CAD build for the part. Positions are in the model's coordinates, mm. A direction names the side the tool comes from. Coordinates: 2 decimals unless noted, no trailing zeros. Loops run counter-clockwise (first coordinate to the right, second up) from the corner with the lowest first, then second, coordinate; pieces in that order, holes last. Notation, with made-up numbers: (80.25, 28.5) -> (101.25, 28.5) arc R28 ccw to (101.25, 55.5) -> close; hole circle Ø11 at (9.5, 43.25). An arc over 180 degrees is marked (long way). Write item = value, one per line. Start each with the question number.
(1) Drill centre lines: line 1 (X direction, y = 49, z = 20.5); line 2 (Y direction, x = 15.24, z = 1.4); line 3 (Z direction, x = 70, y = 14.5). Where is each one in solid material? Low to high. Write a range as from..to.
(2) Pull direction X, two halves, no side cores. Call faces 1 (the face through (51.2, 50.4, 3.8)), 2 (the face through (56.89, 17.223, 6.332)), 3 (the face through (-1.252, 15.328, 59.148)): +X half, -X half, draft (parallel to the pull), parting line (faces both ways), or undercut.
(3) Band-saw the part on C-C (z = 57.15). Write the cut outline in (x, y), and give its area (3 significant figures).
(4) Band-saw the part on D-D (x = 65). Write the cut outline in (y, z) (3 decimals), and give its area (3 significant figures).
(5) Tool access for faces 4 (the face through (1.2, 51.2, 50.4)), 5 (the face through (38, 39, 2.54)), 6 (the face through (4, 10, 76.2)), 7 (the face through (30.28, 1.252, 65.576)), 8 (the face through (5.08, 33, 35)): list every direction of +Z, -Z, +X, -X, +Y, -Y with a clear straight run to the whole face (end or side of a thin tool).
(6) Band-saw the part on A-A (x = 15.24). Count the separate pieces of the cut face and the enclosed holes in it, and give its area (3 significant figures).
(7) Flat gauge pins, fed straight in: P1, Ø6.5, axis at x = 15.24, y = 57.15, coming from the +Z side; P2, Ø3, axis at x = 47.5, z = 25, coming from the +Y side; P3, Ø10, axis at y = 27.5, z = 39.5, coming from the +X side. Where does each tip first touch, or does it go through?
```python
from build123d import *

# Parameters (mm, degrees)
BOSS_EXTRUDE1_DEPTH  = 2.54
BOSS_EXTRUDE2_DEPTH  = 2.54
BOSS_EXTRUDE3_DEPTH  = 2.54
SKETCH6_W            = 2.54
SKETCH6_H            = 76.2
BOSS_EXTRUDE4_DEPTH  = 76.2
CUT_EXTRUDE1_REACH   = 133.982
SKETCH8_W            = 2.54
SKETCH8_H            = 78.74
BOSS_EXTRUDE5_DEPTH  = 76.2
CUT_EXTRUDE2_REACH   = 133.982
SKETCH10_W           = 78.74
SKETCH10_H           = 2.54
BOSS_EXTRUDE6_DEPTH  = 76.2
CUT_EXTRUDE3_REACH   = 133.982
CUT_EXTRUDE5_DEPTH   = 132.982271537
CUT_EXTRUDE6_DEPTH   = 132.982271537
CUT_EXTRUDE9_DEPTH   = 76.2
BOSS_EXTRUDE7_DEPTH  = 7.62
BOSS_EXTRUDE8_DEPTH  = 5.08
BOSS_EXTRUDE9_DEPTH  = 5.08
SKETCH34_R           = 2
CUT_EXTRUDE11_DEPTH  = 12.7
SKETCH35_R           = 2
CUT_EXTRUDE13_DEPTH  = 12.7
SKETCH36_R           = 2
CUT_EXTRUDE14_DEPTH  = 12.7
BOSS_EXTRUDE10_REACH = 133.982
SKETCH37_W           = 25.4
SKETCH37_H           = 25.4
BOSS_EXTRUDE11_REACH = 133.982
SKETCH38_W           = 25.4
SKETCH38_H           = 25.4
SKETCH39_W           = 25.4
SKETCH39_H           = 25.4
BOSS_EXTRUDE12_DEPTH = 5.08


with BuildPart() as part:
    # Sketch1 → Boss-Extrude1 (new body)
    with BuildSketch(Plane.XY):
        Polygon((0, 76.2), (0, 0), (76.2, 0), (76.2, 25.4), (25.4, 76.2), align=None)
    extrude(amount=BOSS_EXTRUDE1_DEPTH)

    # Sketch3 → Boss-Extrude2 (add)
    with BuildSketch(Plane.ZY):
        Polygon((0, 76.2), (25.4, 76.2), (76.2, 25.4), (76.2, 0), (0, 0), align=None)
    extrude(amount=BOSS_EXTRUDE2_DEPTH)

    # Sketch5 → Boss-Extrude3 (add)
    with BuildSketch(Plane.XZ):
        Polygon((-2.54, 76.2), (-2.54, 0), (76.2, 0), (76.2, 25.4), (22.86, 76.2), align=None)
    extrude(amount=BOSS_EXTRUDE3_DEPTH)

    # Sketch6 → Boss-Extrude4 (add)
    with BuildSketch(Plane.XY):
        with Locations((3.81, 38.1)):
            Rectangle(SKETCH6_W, SKETCH6_H)
    extrude(amount=BOSS_EXTRUDE4_DEPTH)

    # Sketch7 → Cut-Extrude1 (cut, up to next)
    with BuildSketch(Plane(origin=(0, 0, 0), x_dir=(0, 0, -1), z_dir=(1, 0, 0)), mode=Mode.PRIVATE) as cut_extrude1_sk1:
        Polygon((-25.4, 76.2), (-76.2, 25.4), (-76.2, 76.2), align=None)
    cut_extrude1_tool1 = extrude(cut_extrude1_sk1.sketch, amount=CUT_EXTRUDE1_REACH, mode=Mode.PRIVATE) & part.part
    add(cut_extrude1_tool1.solids().sort_by_distance((0, 59.266667, 59.266667))[0], mode=Mode.SUBTRACT)

    # Sketch8 → Boss-Extrude5 (add)
    with BuildSketch(Plane(origin=(0, 0, 0), x_dir=(0, 0, -1), z_dir=(1, 0, 0))):
        with Locations((-6.35, 36.83)):
            Rectangle(SKETCH8_W, SKETCH8_H)
    extrude(amount=BOSS_EXTRUDE5_DEPTH)

    # Sketch9 → Cut-Extrude2 (cut, up to next)
    with BuildSketch(Plane.XY, mode=Mode.PRIVATE) as cut_extrude2_sk1:
        Polygon((76.2, 25.4), (25.4, 76.2), (76.2, 76.2), align=None)
    cut_extrude2_tool1 = extrude(cut_extrude2_sk1.sketch, amount=CUT_EXTRUDE2_REACH, mode=Mode.PRIVATE) & part.part
    add(cut_extrude2_tool1.solids().sort_by_distance((59.266667, 59.266667, 0))[0], mode=Mode.SUBTRACT)

    # Sketch10 → Boss-Extrude6 (add)
    with BuildSketch(Plane.XY):
        with Locations((36.83, 3.81)):
            Rectangle(SKETCH10_W, SKETCH10_H)
    extrude(amount=BOSS_EXTRUDE6_DEPTH)

    # Sketch11 → Cut-Extrude3 (cut, up to next)
    with BuildSketch(Plane(origin=(0, 0, 0), x_dir=(1, 0, 0), z_dir=(0, 1, 0)), mode=Mode.PRIVATE) as cut_extrude3_sk1:
        Polygon((22.86, -76.2), (76.2, -25.4), (76.2, -76.2), align=None)
    cut_extrude3_tool1 = extrude(cut_extrude3_sk1.sketch, amount=CUT_EXTRUDE3_REACH, mode=Mode.PRIVATE) & part.part
    add(cut_extrude3_tool1.solids().sort_by_distance((58.42, 0, 59.266667))[0], mode=Mode.SUBTRACT)

    # Sketch12 → Cut-Extrude5 (cut, through all)
    with BuildSketch(Plane(origin=(0, 0, 0), x_dir=(0, 0, -1), z_dir=(1, 0, 0))):
        Polygon((-5.08, 5.08), (-5.08, 2.54), (-7.62, 2.54), (-7.62, 0), (-2.54, 0), (-2.54, 5.08), align=None)
    extrude(amount=CUT_EXTRUDE5_DEPTH, mode=Mode.SUBTRACT)

    # Sketch13 → Cut-Extrude6 (cut, through all)
    with BuildSketch(Plane(origin=(0, 0, 0), x_dir=(1, 0, 0), z_dir=(0, 1, 0))):
        Polygon((0, -2.54), (0, -7.62), (2.54, -7.62), (2.54, -5.08), (5.08, -5.08), (5.08, -2.54), align=None)
    extrude(amount=CUT_EXTRUDE6_DEPTH, mode=Mode.SUBTRACT)

    # Sketch15 → Cut-Extrude9 (cut)
    with BuildSketch(Plane.XY.offset(2.54)):
        Polygon((2.54, 5.08), (0, 5.08), (0, 0), (5.08, 0), (5.08, 2.54), (2.54, 2.54), align=None)
    extrude(amount=CUT_EXTRUDE9_DEPTH, mode=Mode.SUBTRACT)


with BuildPart() as cut_extrude9_piece_1:
    # of the separate pieces the step leaves, piece 1, a body of its own (cut_extrude9_pieces)
    add(part.part.solids().sort_by_distance((0, 0, 2.54))[0])



with BuildPart() as cut_extrude9_piece_2:
    # of the separate pieces the step leaves, piece 2, a body of its own (cut_extrude9_pieces)
    add(part.part.solids().sort_by_distance((2.54, 2.54, 76.2))[0])


with BuildPart() as cut_extrude9_piece_1_1:
    add(cut_extrude9_piece_1.part)

    add(cut_extrude9_piece_2.part)  # Boss-Extrude7 merges Cut-Extrude9 piece 2
    # Sketch17 → Boss-Extrude7 (add)
    with BuildSketch(Plane(origin=(0, 0, 0), x_dir=(-1, 0, 0), z_dir=(0, 0, -1))):
        Polygon((-67.219743879, 34.380256121), (-34.380256121, 67.219743879), (-30.788153673, 63.627641431), (-63.627641431, 30.788153673), align=None)
    extrude(amount=-BOSS_EXTRUDE7_DEPTH)

    # Sketch18 → Boss-Extrude8 (add)
    with BuildSketch(Plane(origin=(0, 0, 0), x_dir=(1, 0, 0), z_dir=(0, 1, 0))):
        Polygon((32.056551724, -67.44137931), (67.003448276, -34.15862069), (63.5, -30.48), (28.553103448, -63.762758621), align=None)
    extrude(amount=BOSS_EXTRUDE8_DEPTH)

    # Sketch19 → Boss-Extrude9 (add)
    with BuildSketch(Plane(origin=(0, 0, 0), x_dir=(0, 0, -1), z_dir=(1, 0, 0))):
        Polygon((-32.545001849, 69.054998151), (-67.219743879, 34.380256121), (-63.627641431, 30.788153673), (-28.9528994, 65.462895703), align=None)
    extrude(amount=BOSS_EXTRUDE9_DEPTH)

    # Sketch34 → Cut-Extrude11 (cut, symmetric)
    with BuildSketch(Plane(origin=(0, 0, 0), x_dir=(0, 0, -1), z_dir=(1, 0, 0))):
        with Locations((-17.78, 57.15)):
            Circle(SKETCH34_R)
        with Locations((-57.15, 15.24)):
            Circle(SKETCH34_R)
    extrude(amount=CUT_EXTRUDE11_DEPTH, both=True, mode=Mode.SUBTRACT)

    # Sketch35 → Cut-Extrude13 (cut, symmetric)
    with BuildSketch(Plane(origin=(0, 0, 0), x_dir=(1, 0, 0), z_dir=(0, 1, 0))):
        with Locations(Location((15.24, -57.15, 0), (0, 0, 270))):
            Circle(SKETCH35_R)
        with Locations(Location((57.15, -17.78, 0), (0, 0, 270))):
            Circle(SKETCH35_R)
    extrude(amount=CUT_EXTRUDE13_DEPTH, both=True, mode=Mode.SUBTRACT)

    # Sketch36 → Cut-Extrude14 (cut, symmetric)
    with BuildSketch(Plane.XY):
        with Locations((57.15, 15.24)):
            Circle(SKETCH36_R)
        with Locations((15.24, 57.15)):
            Circle(SKETCH36_R)
    extrude(amount=CUT_EXTRUDE14_DEPTH, both=True, mode=Mode.SUBTRACT)

    # Boss-Extrude10: up to this face of the body (flat: up to its plane)
    boss_extrude10_end = Plane(cut_extrude9_piece_1_1.part.faces().sort_by_distance((34.248017182, 34.248017182, 7.62))[0])
    # Sketch37 → Boss-Extrude10 (add, up to the picked face)
    with BuildSketch(Plane.XY, mode=Mode.PRIVATE) as boss_extrude10_sk1:
        with Locations((12.7, 12.7)):
            Rectangle(SKETCH37_W, SKETCH37_H)
    boss_extrude10_tool1 = split(extrude(boss_extrude10_sk1.sketch, amount=BOSS_EXTRUDE10_REACH, mode=Mode.PRIVATE), bisect_by=boss_extrude10_end, keep=Keep.BOTH, mode=Mode.PRIVATE)
    add(boss_extrude10_tool1.solids().sort_by(Axis((12.7, 12.7, 0), (0, 0, 1)))[0])

    # Boss-Extrude11: up to this face of the body (flat: up to its plane)
    boss_extrude11_end = Plane(cut_extrude9_piece_1_1.part.faces().sort_by_distance((33.784338957, 5.08, 35.218329504))[0])
    # Sketch38 → Boss-Extrude11 (add, up to the picked face)
    with BuildSketch(Plane(origin=(0, 0, 0), x_dir=(1, 0, 0), z_dir=(0, 1, 0)), mode=Mode.PRIVATE) as boss_extrude11_sk1:
        with Locations((12.7, -15.24)):
            Rectangle(SKETCH38_W, SKETCH38_H)
    boss_extrude11_tool1 = split(extrude(boss_extrude11_sk1.sketch, amount=BOSS_EXTRUDE11_REACH, mode=Mode.PRIVATE), bisect_by=boss_extrude11_end, keep=Keep.BOTH, mode=Mode.PRIVATE)
    add(boss_extrude11_tool1.solids().sort_by(Axis((12.7, 0, 15.24), (0, 1, 0)))[0])

    # Sketch39 → Boss-Extrude12 (add)
    with BuildSketch(Plane(origin=(0, 0, 0), x_dir=(0, 0, -1), z_dir=(1, 0, 0))):
        with Locations((-15.24, 12.7)):
            Rectangle(SKETCH39_W, SKETCH39_H)
    extrude(amount=BOSS_EXTRUDE12_DEPTH)


solid = cut_extrude9_piece_1_1.part
```
Findings below:
q1.line_1 = -2.54..0, 2.54..5.08
q1.line_2 = -2.54..55.15, 59.15..76.2
q1.line_3 = 0..2.54, 5.08..7.62
q2.face_1 = +X half
q2.face_2 = undercut
q2.face_3 = draft
q3.outline = (-2.54, -2.54) -> (13.24, -2.54) -> (13.24, 0) -> (0, 0) -> (0, 13.24) -> (-2.54, 13.24) -> close; (-2.54, 17.24) -> (0, 17.24) -> (0, 37.27) -> (2.54, 37.27) -> (2.54, 17.24) -> (5.08, 17.24) -> (5.08, 44.45) -> (-2.54, 44.45) -> close; (2.54, 2.54) -> (13.24, 2.54) -> (13.24, 5.08) -> (5.08, 5.08) -> (5.08, 13.24) -> (2.54, 13.24) -> close; (17.24, -2.54) -> (42.86, -2.54) -> (42.86, 5.08) -> (17.24, 5.08) -> (17.24, 2.54) -> (35.5, 2.54) -> (35.5, 0) -> (17.24, 0) -> close
q3.area = 427 mm²
q4.outline = (-2.54, 0) -> (36.6, 0) -> (36.6, 7.62) -> (5.08, 7.62) -> (5.08, 36.067) -> (-2.54, 36.067) -> close; hole (0, 2.54) -> (32.161, 2.54) -> (32.161, 5.08) -> (2.54, 5.08) -> (2.54, 32.055) -> (0, 32.055) -> close
q4.area = 365 mm²
q5.face_4 = +Z, +X, -X, +Y
q5.face_5 = none
q5.face_6 = +Z, +X, -X, +Y, -Y
q5.face_7 = +Z
q5.face_8 = +Z, +X, +Y
q6.separate_pieces = 5
q6.enclosed_holes = 0
q6.area = 830 mm²
q7.P1 = 7.62
q7.P2 = 5.08
q7.P3 = 5.08
